Here's how the part is built. I have some questions about the finished solid (model axes, mm). A direction names the side the tool comes from. Round coordinates to 2 decimals unless told otherwise and drop trailing zeros. Write each loop counter-clockwise with the first axis right and the second up, starting at its lowest first coordinate (ties: lowest second). Pieces come first, ordered by that corner, then holes. Notation, with made-up numbers: M 87.25,-26 L 138.25,-26 A8 cw 138.25,-11 Z; hole C -1.75,-11 d1. An arc over 180 degrees is marked long. Use a Markdown table: item, result. Add a question column.
Autodesk Fusion 360 part; units mm, degrees
sketch "Sketch1" plane through (0, 0, -20.5) normal (0, 0, -1) x (-1, 0, 0)
  line L0 (-5, 0) -> (-5, -15)
  line L1 (-5, -15) -> (95, -15)
  line L2 (95, -15) -> (95, 0)
  circle A0 centre (0, -10.5) radius 1
  circle A1 centre (21, -10.5) radius 1
  circle A2 centre (0, 0) radius 7.0711
  line L3 (92, -10.3624) -> (90, -10.3624)
  line L4 (90, -10.3624) -> (90, -2.8871)
  line L5 (90, -2.8871) -> (92, -2.8871)
  line L6 (92, -2.8871) -> (92, -10.3624)
  line L7 (100, 0) -> (42, 0) construction
  line L8 (-5, 15) -> (95, 15)
  line L9 (95, 15) -> (95, 0)
  line L10 (92, 10.3624) -> (90, 10.3624)
  line L11 (92, 2.8871) -> (92, 10.3624)
  line L12 (90, 10.3624) -> (90, 2.8871)
  line L13 (90, 2.8871) -> (92, 2.8871)
  circle A3 centre (21, 10.5) radius 1
  circle A4 centre (0, 10.5) radius 1
  line L14 (-5, 0) -> (-5, 15)
  line L15 (39.3215, 11.0949) -> (49.3215, 11.0949)
  line L16 (49.3215, 11.0949) -> (49.3215, 9.0949)
  line L17 (49.3215, 9.0949) -> (39.3215, 9.0949)
  line L18 (39.3215, 9.0949) -> (39.3215, 11.0949)
  line L19 (54.3215, 11.5) -> (54.3215, -12) construction
  line L20 (54.3215, -11.5) -> (54.3215, 12) construction
  line L21 (49.3215, -11.0949) -> (49.3215, -9.0949)
  line L22 (49.3215, -9.0949) -> (39.3215, -9.0949)
  line L23 (39.3215, -9.0949) -> (39.3215, -11.0949)
  line L24 (39.3215, -11.0949) -> (49.3215, -11.0949)
  line L25 (69.3215, 11.0949) -> (59.3215, 11.0949)
  line L26 (59.3215, 11.0949) -> (59.3215, 9.0949)
  line L27 (59.3215, 9.0949) -> (69.3215, 9.0949)
  line L28 (69.3215, 9.0949) -> (69.3215, 11.0949)
  line L29 (59.3215, -11.0949) -> (59.3215, -9.0949)
  line L30 (69.3215, -9.0949) -> (69.3215, -11.0949)
  line L31 (59.3215, -9.0949) -> (69.3215, -9.0949)
  line L32 (69.3215, -11.0949) -> (59.3215, -11.0949)
  dimension "d1" = 100
  dimension "d3" = 2
  dimension "d4" = 3
  dimension "d77" = 0
  dimension "d78" = 0
  dimension "d79" = 0
  dimension "d80" = 0
  dimension "d93" = 10
  dimension "d94" = 2
  dimension "d95" = 10
extrude "Extrude1" add sketch "Sketch1" along normal blind 2 contours L0 L1 L2 A2 L8 L9 L14
sketch "Sketch2" plane through (0, 0, -22.5) normal (0, 0, -1) x (-1, 0, 0)
  line L0 (25, -6.0704) -> (78.1149, -6.0704)
  arc A0 (78.1149, -6.0704) -> (78.1149, 6.0704) centre (78.1149, 0) ccw
  line L1 (78.1149, 6.0704) -> (25, 6.0704)
  arc A1 (25, 6.0704) -> (25, -6.0704) centre (25, 0) ccw
  line L2 (25, 0) -> (78.1149, 0) construction
extrude "Extrude2" cut sketch "Sketch2" against normal blind 2
fillet "Fillet1" radius 3 6 edges at (5, 15, -21.5) (5, 5, -21.5) (5, -5, -21.5) (5, -15, -21.5) (-95, 15, -21.5) (-95, -15, -21.5)
sketch "Sketch3" plane through (0, 0, -20.5) normal (0, 0, 1) x (1, 0, 0)
sketch "Projection" plane through (0, 0, -20.5) normal (0, 0, 1) x (1, 0, 0)
  line L0 (-25, -6.0704) -> (-78.1149, -6.0704)
  arc A0 (-78.1149, 6.0704) -> (-78.1149, -6.0704) centre (-78.1149, 0) ccw
  line L1 (-78.1149, 6.0704) -> (-25, 6.0704)
  arc A1 (-25, -6.0704) -> (-25, 6.0704) centre (-25, 0) ccw
  line L2 (-92, -2.8871) -> (-90, -2.8871)
  line L3 (-90, -2.8871) -> (-90, -10.3624)
  line L4 (-90, -10.3624) -> (-92, -10.3624)
  line L5 (-92, -10.3624) -> (-92, -2.8871)
  line L6 (-39.3215, -11.0949) -> (-49.3215, -11.0949)
  line L7 (-49.3215, -11.0949) -> (-49.3215, -9.0949)
  line L8 (-49.3215, -9.0949) -> (-39.3215, -9.0949)
  line L9 (-39.3215, -9.0949) -> (-39.3215, -11.0949)
  line L10 (-69.3215, 9.0949) -> (-69.3215, 11.0949)
  line L11 (-69.3215, 11.0949) -> (-59.3215, 11.0949)
  line L12 (-59.3215, 11.0949) -> (-59.3215, 9.0949)
  line L13 (-59.3215, 9.0949) -> (-69.3215, 9.0949)
  circle A2 centre (-21, -10.5) radius 1
  circle A3 centre (-21, 10.5) radius 1
  line L14 (-69.3215, -11.0949) -> (-69.3215, -9.0949)
  line L15 (-69.3215, -9.0949) -> (-59.3215, -9.0949)
  line L16 (-59.3215, -9.0949) -> (-59.3215, -11.0949)
  line L17 (-59.3215, -11.0949) -> (-69.3215, -11.0949)
  line L18 (-90, 2.8871) -> (-92, 2.8871)
  line L19 (-92, 2.8871) -> (-92, 10.3624)
  line L20 (-92, 10.3624) -> (-90, 10.3624)
  line L21 (-90, 10.3624) -> (-90, 2.8871)
  circle A4 centre (0, 10.5) radius 1
  line L22 (-39.3215, 9.0949) -> (-49.3215, 9.0949)
  line L23 (-49.3215, 9.0949) -> (-49.3215, 11.0949)
  line L24 (-49.3215, 11.0949) -> (-39.3215, 11.0949)
  line L25 (-39.3215, 11.0949) -> (-39.3215, 9.0949)
  circle A5 centre (0, -10.5) radius 1
  arc A6 (-95, -12) -> (-92, -15) centre (-92, -12) ccw
  line L26 (-92, -15) -> (2, -15)
  arc A7 (2, -15) -> (5, -12) centre (2, -12) ccw
  line L27 (5, -12) -> (5, -9.8705)
  arc A8 (5, -9.8705) -> (1.4042, -6.9302) centre (2, -9.8705) ccw
  arc A9 (1.4042, 6.9302) -> (1.4042, -6.9302) centre (0, 0) ccw
  arc A10 (1.4042, 6.9302) -> (5, 9.8705) centre (2, 9.8705) ccw
  line L28 (5, 9.8705) -> (5, 12)
  arc A11 (5, 12) -> (2, 15) centre (2, 12) ccw
  line L29 (2, 15) -> (-92, 15)
  arc A12 (-92, 15) -> (-95, 12) centre (-92, 12) ccw
  line L30 (-95, 12) -> (-95, -12)
equation "thiccness = 2 mm"
equation "d3 = thiccness"
equation "d11 = thiccness"
equation "d94 = thiccness"
Item 1: I need wall thicknesses on probe 1 along Y at (x, z) = (0, -21.15); probe 2 along Y at (x, z) = (-67.5, -21.1); probe 3 along Y at (x, z) = (-72, -21.55). Which ranges of each line are inside material? Lowest first, please. Write a range as from..to.
Item 2: For pin 1 Ø12 at (x, y) = (-55, -3) entering from -Z, with a flat end and sliding along its axis, tell me the tip position at first contact or that it passes through.
Item 3: On a 3-axis mill with a long thin cutter (end or side, diameter ignored), from which of +Z, -Z, +X, -X, +Y, -Y can I reach the whole of each face in a straight line? I mean faces 1 (the face through (-44, -9.095, -21)), 2 (the face through (5, -11, -21)). Say none if no direction works.
Item 4: Imagine slicing it at B-B on x = 0. List the corners of the cut face in (y, z) for me.
Item 5: Imagine slicing it at A-A on y = 0. List the corners of the cut face in (x, z) for me.
Item 6: Imagine slicing it at D-D on x = -21. List the corners of the cut face in (y, z) for me, plus the area to 3 significant figures.
Item 7: Imagine slicing it at C-C on y = -8. List the corners of the cut face in (x, z) for me.
Item 8: If we mould it in two halves opening along Y, with no side actions, what happens to faces 3 (the face through (-44, -11.095, -21)), 4 (the face through (-95, 0, -21)), 5 (the face through (-44, -15, -21)), 6 (the face through (-39.322, -10, -21))? For each: +Y half, -Y half, draft (parallel to the pull), parting line (faces both ways), or undercut.
The answers:
| question | item | result |
|---|---|---|
| 1 | probe 1 | -15..-11.5, -9.5..-7.07, 7.07..9.5, 11.5..15 |
| 1 | probe 2 | -15..-11.09, -9.09..-6.07, 6.07..9.09, 11.09..15 |
| 1 | probe 3 | -15..-6.07, 6.07..15 |
| 2 | pin 1 | z = -22.5 |
| 3 | face 1 | +Z, -Z |
| 3 | face 2 | +Z, -Z, +X, +Y, -Y |
| 4 | outline | M -15,-22.5 L -11.5,-22.5 L -11.5,-20.5 L -15,-20.5 Z; M -9.5,-22.5 L -7.07,-22.5 L -7.07,-20.5 L -9.5,-20.5 Z; M 7.07,-22.5 L 9.5,-22.5 L 9.5,-20.5 L 7.07,-20.5 Z; M 11.5,-22.5 L 15,-22.5 L 15,-20.5 L 11.5,-20.5 Z |
| 5 | outline | M -95,-22.5 L -84.19,-22.5 L -84.19,-20.5 L -95,-20.5 Z; M -18.93,-22.5 L -7.07,-22.5 L -7.07,-20.5 L -18.93,-20.5 Z |
| 6 | outline | M -15,-22.5 L -11.5,-22.5 L -11.5,-20.5 L -15,-20.5 Z; M -9.5,-22.5 L -4.57,-22.5 L -4.57,-20.5 L -9.5,-20.5 Z; M 4.57,-22.5 L 9.5,-22.5 L 9.5,-20.5 L 4.57,-20.5 Z; M 11.5,-22.5 L 15,-22.5 L 15,-20.5 L 11.5,-20.5 Z |
| 6 | area | 33.7 mm² |
| 7 | outline | M -95,-22.5 L -92,-22.5 L -92,-20.5 L -95,-20.5 Z; M -90,-22.5 L 4.35,-22.5 L 4.35,-20.5 L -90,-20.5 Z |
| 8 | face 3 | undercut |
| 8 | face 4 | draft |
| 8 | face 5 | -Y half |
| 8 | face 6 | undercut |
